Autodesk Inventor part; units mm, degrees
ref_plane "YZ Plane" through (0, 0, 0) normal (1, 0, 0) x (0, 1, 0)
ref_plane "XZ Plane" through (0, 0, 0) normal (0, 1, 0) x (-1, 0, 0)
ref_plane "XY Plane" through (0, 0, 0) normal (0, 0, 1) x (1, 0, 0)
sketch "Sketch10" plane through (0, 0, 0) normal (0, 1, 0) x (-1, 0, 0)
  circle A0 centre (0, 0) radius 12.25
  dimension "d115" = 24.5
extrude "Extrusion8" add sketch "Sketch10" along normal blind 2.7
sketch "Sketch15" plane through (0, 0, 0) normal (0, -1, 0) x (1, 0, 0)
  circle A0 centre (0, 0) radius 12.75 construction
  line L0 (12.75, 0) -> (0, 0) construction
  line L1 (0, 0) -> (-11.5554, -5.3884) construction
  line L2 (0, 0) -> (-11.5554, 5.3884) construction
  circle A1 centre (-11.5554, -5.3884) radius 1.375
  circle A2 centre (12.75, 0) radius 1.375
  circle A3 centre (-11.5554, 5.3884) radius 1.375
  dimension "d116" = 25.5
  dimension "d117" = 25
  dimension "d118" = 25
  dimension "d119" = 2.75
extrude "Extrusion13" cut sketch "Sketch15" against normal up to surface (2.7 mm away)
sketch "Sketch17" plane through (0, 2.7, 0) normal (0, 1, 0) x (1, 0, 0)
  line L0 (-3.885, 10.76) -> (2.615, 10.76)
  line L1 (2.615, 10.76) -> (2.615, 8.16)
  line L2 (2.615, 8.16) -> (-3.885, 8.16)
  line L3 (-3.885, 8.16) -> (-3.885, 10.76)
  line L4 (2.615, 8.16) -> (-3.885, 10.76) construction
  line L5 (-3.885, 8.16) -> (2.615, 10.76) construction
  point P0 (0, 0)
  point P1 (-0.635, 9.46)
  dimension "d130" = 2.6
  dimension "d131" = 6.5
  dimension "d144" = 9.46
  dimension "d145" = 0.635
extrude "Extrusion14" cut sketch "Sketch17" against normal up to next
sketch "Sketch11" plane through (0, 0, 0) normal (0, -1, 0) x (1, 0, 0)
  line L0 (7.5, -7.7326) -> (-7.5, -7.7326)
  line L1 (-7.5, -7.7326) -> (-7.5, 12.25)
  line L2 (-7.5, 12.25) -> (7.5, 12.25)
  line L3 (7.5, 12.25) -> (7.5, -7.7326)
  arc A0 (12.1857, 1.2539) -> (12.1857, -1.2539) centre (12.75, 0) ccw
  arc A1 (-10.5141, -6.2863) -> (12.1857, -1.2539) centre (0, 0) ccw
  arc A2 (-10.5141, -6.2863) -> (-11.5739, -4.0135) centre (-11.5554, -5.3884) ccw
  arc A3 (-11.5739, 4.0135) -> (-11.5739, -4.0135) centre (0, 0) ccw
  arc A4 (-11.5739, 4.0135) -> (-10.5141, 6.2863) centre (-11.5554, 5.3884) ccw
  arc A5 (12.1857, 1.2539) -> (-10.5141, 6.2863) centre (0, 0) ccw
  dimension "d78" = 15
  dimension "d122" = 7.5
extrude "Extrusion9" cut sketch "Sketch11" against normal blind 1.54 contours L0 L1 A5 L3 | A5 L2 L3 | L1 L2 A5
ref_plane "Work Plane4" through (0, 0, -12.25) normal (0, 0, -1) x (-1, 0, 0)
ref_plane "Work Plane3" through (0, 0, -7.7326) normal (-1, 0, 0) x (0, 0, 1)
sketch "Sketch13" plane through (0, 0, -12.25) normal (0, 0, -1) x (-1, 0, 0)
  line L0 (-7.5, 1.54) -> (-7.5, 0)
  line L1 (-12.1857, 0) -> (-7.5, 0)
  line L2 (-12.1857, 0) -> (-12.1857, 2.7)
  line L3 (10.5141, 2.7) -> (-12.1857, 2.7)
  line L4 (10.5141, 2.7) -> (10.5141, 0)
  line L5 (7.5, 0) -> (10.5141, 0)
  line L6 (7.5, 0) -> (7.5, 1.54)
  line L7 (7.5, 1.54) -> (-7.5, 1.54)
  line L8 (7.5, 0) -> (7.5, -1.6588)
  line L9 (7.5, -1.6588) -> (9.3, -1.6588)
  line L10 (9.3, -1.6588) -> (8.4, -0.1)
  line L11 (8.4, -0.1) -> (8.4, 0)
  line L12 (7.5, 0) -> (8.4, 0)
  line L13 (7.5, 0) -> (10.5141, 0)
  point P0 (0, 15)
  dimension "d146" = 0.9
  dimension "d147" = 60
  dimension "d148" = 1.8
  dimension "d149" = 0.1
extrude "Extrusion11" add sketch "Sketch13" against normal blind 18.4 contours L5 L11 L10 L9 L8
mirror "Mirror1" about plane through (0, 0, -7.7326) normal (-1, 0, 0) of "Extrusion11"
sketch "Sketch14" plane through (0, 0, 0) normal (0, -1, 0) x (1, 0, 0)
  circle A0 centre (0, 0) radius 12.25
  arc A1 (7.5, 9.6857) -> (-7.5, 9.6857) centre (0, 0) ccw
  circle A2 centre (0, 0) radius 24.8523
  point P0 (1.5155, -12.4)
extrude "Extrusion12" cut sketch "Sketch14" along normal up to next
sketch "Sketch19" plane through (0, 0, 0) normal (0, -1, 0) x (1, 0, 0)
  arc A0 (-7.5, -8.3853) -> (7.5, -8.3853) centre (0, 0) ccw
  arc A1 (-7.5, -9.6857) -> (7.5, -9.6857) centre (0, 0) ccw
  line L0 (-7.5, -9.6857) -> (-7.5, 6.15)
  line L1 (7.5, -9.6857) -> (7.5, 6.15)
  point P0 (-7.5, -9.8747)
  point P1 (7.5, -9.8747)
  point P2 (-7.5, -9.7488)
  point P3 (7.5, -9.7488)
  dimension "d141" = 1
extrude "Extrusion15" add sketch "Sketch19" along normal up to surface (1.6588 mm away)
sketch "Sketch21" plane through (0, 1.54, 0) normal (0, -1, 0) x (1, 0, 0)
  circle A0 centre (0, 11) radius 0.5
  point P0 (0, 0)
  dimension "d154" = 11
  dimension "d155" = 1
extrude "Extrusion17" cut sketch "Sketch21" against normal blind 0.25
fillet "Fillet1" radius 0.25 2 edges at (-0.5, 1.79, 11) (-0.5, 1.54, 11)
sketch "Sketch22" plane through (0, -1.6588, 0) normal (0, -1, 0) x (1, 0, 0)
  arc A0 (-7.3, -9.8373) -> (7.3, -9.8373) centre (0, 0) ccw
  arc A1 (-7.3, -8.5599) -> (7.3, -8.5599) centre (0, 0) ccw
  line L0 (-7.3, -8.5599) -> (-7.3, -9.8373)
  line L1 (7.3, -8.5599) -> (7.3, -9.8373)
  arc A2 (-9.3, -7.9732) -> (-7.5, -9.6857) centre (0, 0) ccw
  arc A3 (-7.5, -9.6857) -> (7.5, -9.6857) centre (0, 0) ccw
  arc A4 (7.5, -9.6857) -> (9.3, -7.9732) centre (0, 0) ccw
  line L2 (9.3, -7.9732) -> (9.3, 6.15)
  line L3 (9.3, 6.15) -> (7.5, 6.15)
  line L4 (7.5, -8.3853) -> (7.5, 6.15)
  arc A5 (-7.5, -8.3853) -> (7.5, -8.3853) centre (0, 0) ccw
  line L5 (-7.5, -8.3853) -> (-7.5, 6.15)
  line L6 (-9.3, 6.15) -> (-7.5, 6.15)
  line L7 (-9.3, -7.9732) -> (-9.3, 6.15)
  arc A6 (-7.5, -8.3853) -> (7.5, -8.3853) centre (0, 0) ccw
  arc A7 (7.5, -9.6857) -> (9.3, -7.9732) centre (0, 0) ccw
  dimension "d163" = 0.2
  dimension "d164" = 0.2
extrude "Extrusion18" add sketch "Sketch22" along normal blind 3.018 contours L0 A1 L1 A0
sketch "Sketch23" plane through (0, 0, 0) normal (0, -1, 0) x (1, 0, 0)
  arc A0 (-7.3, -8.5599) -> (7.3, -8.5599) centre (0, 0) ccw
  line L0 (-5.3558, -9.8933) -> (5.3558, -9.8933)
  line L1 (2.615, -10.76) -> (-3.284, -10.76)
  line L2 (-3.885, -8.16) -> (2.615, -8.16)
  dimension "d165" = 0.8667
  dimension "d166" = 2.6
extrude "Extrusion19" add sketch "Sketch23" along normal blind 1
properties part number "bottom2_2" material "Acrylic"
Geometry check sheet. Reference: the model listing, model coordinates, mm. A direction names the side the tool comes from. Round coordinates to 2 decimals unless told otherwise and drop trailing zeros. Loops run counter-clockwise (first coordinate to the right, second up) from the corner with the lowest first, then second, coordinate; pieces in that order, holes last.
Item 1: Cross-section at A-A on y = 2.25. Record the boundary of the cut face in (x, z) (3 decimals).
Item 2: Cross-section at C-C on z = 2. Record the boundary of the cut face in (x, y), then the cut area to 3 significant figures.
Item 3: Cross-section at B-B on x = -2. Record the boundary of the cut face in (y, z), then the cut area to 3 significant figures.
Item 4: Thickness scan on line 1 (Y direction, x = -2.75, z = 10.5); line 2 (Y direction, x = -1.75, z = -10); line 3 (X direction, y = 2.25, z = 0) (3 decimals). Record the ranges inside material, lowest first.
Item 5: Access from +Z, -Z, +X, -X, +Y, -Y to the whole of each face (thin tool, end or side, straight path). Record for faces 5 (the flat face through (8.844, -0.868, -1.489)), 6 (the flat face through (7.5, 0, 1)), 7 (the flat face through (-7.3, -3, -9)), 8 (the flat face through (-8, -1, 6.15)).
Item 6: Cross-section at D-D on x = 7. Record the boundary of the cut face in (y, z), then the cut area to 3 significant figures.
Item 7: Gauge pin test, flat ends, axial feed: pin 1 (1.6 mm diameter, centred on x = 8, z = -5.5, fed in from -Y); pin 2 (1.1 mm diameter, centred on x = -0.5, y = -0.5, fed in from +Z); pin 3 (1.4 mm diameter, centred on x = -10.5, z = -4, fed in from -Y). Record the tip position at first contact, or that the pin passes through.
Item 8: Mould release check, pull along X, two halves, no side actions. Record for faces 1 (the flat face through (2.615, 1, -9)), 2 (the flat face through (0, -4.677, -11.5)), 3 (the flat face through (-0.1, -0.5, -9.893)), 4 (the flat face through (7.3, -3, -9)): pulls with the +X half, pulls with the -X half, needs draft (parallel to the pull), parting line crosses it, or undercut.
Answer sheet:
1. outline: (-11.574, -4.014) arc R1.375 cw to (-10.514, -6.286) arc R12.25 ccw to (12.186, -1.254) arc R1.375 cw to (12.186, 1.254) arc R12.25 ccw to (-10.514, 6.286) arc R1.375 cw to (-11.574, 4.014) arc R12.25 ccw to start; hole (-3.885, -10.76) - (2.615, -10.76) - (2.615, -8.16) - (-3.885, -8.16) - close
2. outline: (-12.09, 0) - (-8.4, 0) - (-8.4, -0.1) - (-9.3, -1.66) - (-7.5, -1.66) - (-7.5, 1.54) - (7.5, 1.54) - (7.5, -1.66) - (9.3, -1.66) - (8.4, -0.1) - (8.4, 0) - (12.09, 0) - (12.09, 2.7) - (-12.09, 2.7) - close
2. area: 46.6 mm2
3. outline: (-4.68, -12.09) - (0, -12.09) - (2.7, -12.09) - (2.7, -10.76) - (0, -10.76) - (0, -9.89) - (-1, -9.89) - (-1, -11.07) - (-4.68, -11.07) - close; (0, -8.16) - (2.7, -8.16) - (2.7, 12.09) - (1.54, 12.09) - (1.54, -7.73) - (0, -7.73) - close
3. area: 33.6 mm2
4. line 1: y = 1.54 to 2.7
4. line 2: y = -1 to 0
4. line 3: x = -12.25 to 11.375
5. face 5: +Z, -Z, +X
5. face 6: +Z, -Y
5. face 7: +Z, -Z, -X, -Y
5. face 8: +Z, +X, -X, -Y
6. outline: (-4.68, -10.05) - (0, -10.05) - (2.7, -10.05) - (2.7, 10.05) - (1.54, 10.05) - (1.54, -7.73) - (0, -7.73) - (0, -8.81) - (-4.68, -8.81) - close
6. area: 32.7 mm2
7. pin 1: stops at y = -1.66
7. pin 2: stops at z = -7.73
7. pin 3: stops at y = 0
8. face 1: undercut
8. face 2: needs draft
8. face 3: undercut
8. face 4: pulls with the +X half
